Input: part model. Units: mm. Frame: model coordinates. A direction names the side the tool comes from. Give positions to 0.01 mm unless a question says otherwise; leave off trailing zeros. Loops run counter-clockwise (first coordinate to the right, second up) from the corner with the lowest first, then second, coordinate; pieces in that order, holes last. Notation, with made-up numbers: M -16,48 L 7,48 A10 ccw 7,58 Z; hole C 0.5,-10 d6. An arc over 180 degrees is marked long. One line per item, written item: value. Start each with the question number.
(1) Pin query (flat end, axial travel): P1, Ø5, axis at y = -18.5, z = 683.5, coming from the +X side; P2, Ø1, axis at x = -1.5, y = 15.5, coming from the -Z side; P3, Ø1.6, axis at x = -1.5, z = 670, coming from the +Y side. Return the tip coordinate at first contact, or that it passes through.
(2) Section D-D on z = 710. Output: boundary loops of the cut face in (x, y) (3 decimals), plus the area to 3 significant figures.
(3) Section C-C on y = -11.5. Output: boundary loops of the cut face in (x, z) (3 decimals).
(4) Access query for faces 1 (the flat face through (-2, 48, 618.102)), 2 (the flat face through (-2, 20, 734.927)), 3 (the flat face through (-2, 20, 601.277)). Directions: +Z, -Z, +X, -X, +Y, -Y. A direction counts if a zero-diameter tool reaches every point of the face in a straight line with its end or side. Return the directions, or none.
(5) Pull-direction query (Y, two-part tool) for faces 4 (the flat face through (-2, 48, 638.102)), 5 (the flat face through (-2, 46.825, 628)), 6 (the flat face through (-2, -50, 728)), 7 (the cylindrical face through (-1.565, 0.66, 633.116)); classes: released by +Y, released by -Y, zero draft, split by the parting line, or undercut.
(6) Section A-A on z = 607. Output: boundary loops of the cut face in (x, y) (3 decimals), plus the area to 3 significant figures.
(7) Section B-B on y = 7. Output: boundary loops of the cut face in (x, z) (3 decimals).
(8) Ray query, line 1 along Z through (x, y) = (-0.4, 0); line 2 along Y through (x, z) = (-1.8, 604); line 3 along Z through (x, y) = (-0.9, -4.5). Return the intervals inside material, ascending. Write a range as from..to.
```python
from build123d import *

# Parameters (mm, degrees)
SKETCH46_W           = 140
SKETCH46_H           = 99.999981374
SKETCH46_R           = 15
SKETCH46_W_2         = 21.745
SKETCH46_H_2         = 23.125
BOSS_EXTRUDE11_DEPTH = 3.175
SKETCH47_W           = 3.175
SKETCH47_H           = 20
SKETCH47_W_2         = 20
SKETCH47_H_2         = 3.175
CUT_EXTRUDE23_DEPTH  = 3.175


with BuildPart() as part:
    # Sketch46 → Boss-Extrude11 (new body)
    with BuildSketch(Plane.ZY):
        with Locations((668.101928689, 4.4643e-05)):
            Rectangle(SKETCH46_W, SKETCH46_H)
        with Locations((648.101928689, 4.4643e-05)):
            Circle(SKETCH46_R, mode=Mode.SUBTRACT)
        with Locations((614.504428689, -8.437455357)):
            Rectangle(SKETCH46_W_2, SKETCH46_H_2, mode=Mode.SUBTRACT)
    extrude(amount=BOSS_EXTRUDE11_DEPTH)

    # Sketch47 → Cut-Extrude23 (cut)
    with BuildSketch(Plane.ZY.offset(3.175)):
        with Locations((736.514428689, -19.99996467)):
            Rectangle(SKETCH47_W, SKETCH47_H)
        with Locations((736.514428689, 20.00003533)):
            Rectangle(SKETCH47_W, SKETCH47_H)
        with Locations((599.689428689, -19.99996467)):
            Rectangle(SKETCH47_W, SKETCH47_H)
        with Locations((599.689428689, 20.00003533)):
            Rectangle(SKETCH47_W, SKETCH47_H)
        with Locations((668.101928689, 48.41253533)):
            Rectangle(SKETCH47_W_2, SKETCH47_H_2)
        with Locations((708.101928689, 48.41253533)):
            Rectangle(SKETCH47_W_2, SKETCH47_H_2)
        with Locations((628.101928689, 48.41253533)):
            Rectangle(SKETCH47_W_2, SKETCH47_H_2)
        with Locations((668.101928689, -48.412446044)):
            Rectangle(SKETCH47_W_2, SKETCH47_H_2)
        with Locations((708.101928689, -48.412446044)):
            Rectangle(SKETCH47_W_2, SKETCH47_H_2)
        with Locations((628.101928689, -48.412446044)):
            Rectangle(SKETCH47_W_2, SKETCH47_H_2)
    extrude(amount=-CUT_EXTRUDE23_DEPTH, mode=Mode.SUBTRACT)


solid = part.part
```
Output values:
1. P1: stops at x = 0
1. P2: stops at z = 601.28
1. P3: stops at y = 46.83
2. outline: M -3.175,-46.825 L 0,-46.825 L 0,46.825 L -3.175,46.825 Z
2. area: 297 mm²
3. outline: M -3.175,601.277 L 0,601.277 L 0,603.632 L -3.175,603.632 Z; M -3.175,625.377 L 0,625.377 L 0,638.471 L -3.175,638.471 Z; M -3.175,657.733 L 0,657.733 L 0,734.927 L -3.175,734.927 Z
4. face 1: +X, -X, +Y
4. face 2: +Z, +X, -X
4. face 3: -Z, +X, -X
5. face 4: zero draft
5. face 5: released by +Y
5. face 6: released by -Y
5. face 7: undercut
6. outline: M -3.175,-50 L 0,-50 L 0,-20 L -3.175,-20 Z; M -3.175,3.125 L 0,3.125 L 0,50 L -3.175,50 Z
6. area: 244 mm²
7. outline: M -3.175,598.102 L 0,598.102 L 0,634.835 L -3.175,634.835 Z; M -3.175,661.368 L 0,661.368 L 0,738.102 L -3.175,738.102 Z
8. line 1: z = 598.1..603.63, 625.38..633.1, 663.1..738.1
8. line 2: y = -50..-20, 3.13..50
8. line 3: z = 598.1..603.63, 625.38..633.79, 662.41..738.1
